CAD build for the part. Positions are in the model's coordinates, mm. A direction names the side the tool comes from. Round coordinates to 2 decimals unless told otherwise and drop trailing zeros. Write each loop counter-clockwise with the first axis right and the second up, starting at its lowest first coordinate (ties: lowest second). Pieces come first, ordered by that corner, then holes. Notation, with made-up numbers: (24, 66) - (30, 66) arc R27 ccw to (30, 102) - close; hole circle Ø4 at (28.25, 74.25). An arc over 180 degrees is marked (long way). Put each result on its own line as item: value. Start each with the question number.
Item 1: Mould opens along Z. For faces 1 (the flat face through (17, 8, 0)), 2 (the cylindrical face through (8.619, -7.656, -1.005)), 3 (the flat face through (40, 20.1, 0)), 4 (the cylindrical face through (7.71, 1.93, -2.52)) say: released by +Z, released by -Z, zero draft, split by the parting line, or undercut.
Item 2: Pin check, flat tips, straight feed: pin 1 Ø6 at (x, z) = (94, 2) entering from -Y; pin 2 Ø7 at (x, z) = (39.5, -1) entering from +Y; pin 3 Ø12 at (x, z) = (20.5, -14.5) entering from +Y; pin 4 Ø4 at (x, z) = (90, 0) entering from +Y. Stop position of each tip, or through.
Item 3: Cut at B-B (z = 0). Give the cut face in (x, y) (3 decimals).
Item 4: 3-axis set-ups, long thin cutter, end or side, ignore diameter. For faces 5 (the cylindrical face through (43.1, 27.81, 0.69)), 6 (the cylindrical face through (83.9, 12.4, 6.5)), 7 (the flat face through (15.2, 0, 0)): which of +Z, -Z, +X, -X, +Y, -Y reach the whole face in a straight line?
Item 5: Cut at C-C (x = 40). Give the cut face in (y, z) (3 decimals).
Item 6: Drill centre lines: line 1 (Y direction, x = 3.5, z = 0) (3 decimals); line 2 (X direction, y = 29, z = 0) (3 decimals). Where is each one in solid material? Low to high. Write a range as from..to.
Item 7: Cut at A-A (y = 0). Give the cut face in (x, z) (3 decimals), and give its area (3 significant figures).
Item 8: Cut at D-D (y = 24). Give the cut face in (x, z) (3 decimals), and give its area (3 significant figures).
```python
from build123d import *

# Parameters (mm, degrees)
BODY_SKETCH_W          = 45
BODY_SKETCH_H          = 36.6
BODY_DEPTH             = 20.3
INLET_SKETCH_W         = 17
INLET_SKETCH_H         = 7.722
SPRING_CAP_SKETCH_W    = 43.2
SPRING_CAP_SKETCH_H    = 14
OUTLET_SKETCH_W        = 7.722
OUTLET_SKETCH_H        = 17
INLET_SOCKET_SKETCH_W  = 16.2
INLET_SOCKET_SKETCH_H  = 3.175
OUTLET_SOCKET_SKETCH_W = 3.175
OUTLET_SOCKET_SKETCH_H = 16.2


with BuildPart() as part:
    # Body Sketch → Body (new, symmetric)
    with BuildSketch(Plane.XY):
        with Locations((39.5, 0)):
            Rectangle(BODY_SKETCH_W, BODY_SKETCH_H)
    extrude(amount=BODY_DEPTH, both=True)

    # Inlet Sketch → Inlet (revolve)
    with BuildSketch(Plane.XY, mode=Mode.PRIVATE) as inlet_sk:
        with Locations((8.5, 3.861)):
            Rectangle(INLET_SKETCH_W, INLET_SKETCH_H)
    revolve(inlet_sk.sketch.rotate(Axis((-1000, 0, 0), (1, 0, 0)), 90), axis=Axis((-1000, 0, 0), (1, 0, 0)))

    # Spring Cap Sketch → Spring Cap (revolve)
    with BuildSketch(Plane.XY, mode=Mode.PRIVATE) as spring_cap_sk:
        with Locations((83.6, 7)):
            Rectangle(SPRING_CAP_SKETCH_W, SPRING_CAP_SKETCH_H)
    revolve(spring_cap_sk.sketch.rotate(Axis((-1000, 0, 0), (1, 0, 0)), 90), axis=Axis((-1000, 0, 0), (1, 0, 0)))

    # Outlet Sketch → Outlet (revolve)
    with BuildSketch(Plane.XY, mode=Mode.PRIVATE) as outlet_sk:
        with Locations((43.861, 26.8)):
            Rectangle(OUTLET_SKETCH_W, OUTLET_SKETCH_H)
    revolve(outlet_sk.sketch.rotate(Axis((40, 0, 0), (0, 1, 0)), 90), axis=Axis((40, 0, 0), (0, 1, 0)))

    # Inlet Socket Sketch → Inlet Socket (revolve, cut)
    with BuildSketch(Plane.XY, mode=Mode.PRIVATE) as inlet_socket_sk:
        with Locations((7.1, 1.5875)):
            Rectangle(INLET_SOCKET_SKETCH_W, INLET_SOCKET_SKETCH_H)
    revolve(inlet_socket_sk.sketch.rotate(Axis((-1000, 0, 0), (1, 0, 0)), 90), axis=Axis((-1000, 0, 0), (1, 0, 0)), mode=Mode.SUBTRACT)

    # Outlet Socket Sketch → Outlet Socket (revolve, cut)
    with BuildSketch(Plane.XY, mode=Mode.PRIVATE) as outlet_socket_sk:
        with Locations((41.5875, 28.2)):
            Rectangle(OUTLET_SOCKET_SKETCH_W, OUTLET_SOCKET_SKETCH_H)
    revolve(outlet_socket_sk.sketch.rotate(Axis((40, 0, 0), (0, 1, 0)), 90), axis=Axis((40, 0, 0), (0, 1, 0)), mode=Mode.SUBTRACT)


solid = part.part
```
Output values:
1. face 1: zero draft
1. face 2: split by the parting line
1. face 3: undercut
1. face 4: undercut
2. pin 1: y = -14
2. pin 2: y = 35.3
2. pin 3: y = 18.3
2. pin 4: y = 14
3. outline: (0, -7.722) - (17, -7.722) - (17, -18.3) - (62, -18.3) - (62, -14) - (105.2, -14) - (105.2, 14) - (62, 14) - (62, 18.3) - (47.722, 18.3) - (47.722, 35.3) - (43.175, 35.3) - (43.175, 20.1) - (36.825, 20.1) - (36.825, 35.3) - (32.278, 35.3) - (32.278, 18.3) - (17, 18.3) - (17, 7.722) - (0, 7.722) - (0, 3.175) - (15.2, 3.175) - (15.2, -3.175) - (0, -3.175) - close
4. face 5: +Y
4. face 6: +X
4. face 7: -X
5. outline: (-18.3, -20.3) - (18.3, -20.3) - (18.3, -7.722) - (35.3, -7.722) - (35.3, -3.175) - (20.1, -3.175) - (20.1, 3.175) - (35.3, 3.175) - (35.3, 7.722) - (18.3, 7.722) - (18.3, 20.3) - (-18.3, 20.3) - close
6. line 1: -7.722..-3.175, 3.175..7.722
6. line 2: 32.278..36.825, 43.175..47.722
7. outline: (0, -7.722) - (17, -7.722) - (17, -20.3) - (62, -20.3) - (62, -14) - (105.2, -14) - (105.2, 14) - (62, 14) - (62, 20.3) - (17, 20.3) - (17, 7.722) - (0, 7.722) - (0, 3.175) - (15.2, 3.175) - (15.2, -3.175) - (0, -3.175) - close
7. area: 3,200 mm2
8. outline: circle Ø15.444 at (40, 0); hole circle Ø6.35 at (40, 0)
8. area: 156 mm2
